Read the model definition and answer for the solid it produces. Units are mm, in the model's axes. Round coordinates to 2 decimals unless told otherwise and drop trailing zeros. Loops run counter-clockwise (first coordinate to the right, second up) from the corner with the lowest first, then second, coordinate; pieces in that order, holes last. Notation, with made-up numbers: (40.5, -31) - (77.5, -31) arc R16 cw to (77.5, 0) - close; hole circle Ø1 at (89.5, 17). An arc over 180 degrees is marked (long way). Use CSV: the item, a comma, the result in double quotes. Start each with the question number.
1. Consider line 1 along X through (y, z) = (-41, 2.55); line 2 along X through (y, z) = (-29.5, 1.7); line 3 along Y through (x, z) = (180.5, 0.3). Determine where each line is inside the solid, lowest interval first.
2. Given pin 1 Ø2.5 at (x, z) = (28, 1.5) entering from -Y; pin 2 Ø2.5 at (x, y) = (-193.01, -130.08) entering from -Z, each flat-ended and moving along its own axis, determine where each tip first touches the part or whether it passes through.
3. Find section A-A (z = 4). State how many separate pieces and enclosed holes the cut face has, and give its area (3 significant figures).
4. Find section B-B (x = -120.5). Give the vertices of the cut face in (y, z), and give its area (3 significant figures).
from build123d import *

# Parameters (mm, degrees)
SKETCH1_W           = 557
SKETCH1_H           = 150
BOSS_EXTRUDE1_DEPTH = 5
SKETCH2_W           = 30
SKETCH2_H           = 10.4
BOSS_EXTRUDE2_DEPTH = 5
SKETCH3_R           = 2.1
CUT_EXTRUDE1_DEPTH  = 10
SKETCH4_R           = 2.1
CUT_EXTRUDE2_DEPTH  = 10
SKETCH5_R           = 2.1
CUT_EXTRUDE3_DEPTH  = 10
SKETCH6_R           = 2.1
CUT_EXTRUDE4_DEPTH  = 10


with BuildPart() as part:
    # Sketch1 → Boss-Extrude1 (new body)
    with BuildSketch(Plane.XY):
        with Locations((-17.512478204, -80.075206465)):
            Rectangle(SKETCH1_W, SKETCH1_H)
    extrude(amount=BOSS_EXTRUDE1_DEPTH)

    # Sketch2 → Boss-Extrude2 (add)
    with BuildSketch(Plane.XY.offset(5)):
        with Locations((-156.762478204, -155.075206465)):
            Rectangle(SKETCH2_W, SKETCH2_H)
        with Locations((121.737521796, -155.075206465)):
            Rectangle(SKETCH2_W, SKETCH2_H)
    extrude(amount=-BOSS_EXTRUDE2_DEPTH)

    # Sketch3 → Cut-Extrude1 (cut)
    with BuildSketch(Plane.XY.offset(5)):
        with Locations((-276.012478204, -28.705206465)):
            Circle(SKETCH3_R)
        with Locations((-276.012478204, -42.775206465)):
            Circle(SKETCH3_R)
        with Locations((240.987521796, -42.775206465)):
            Circle(SKETCH3_R)
        with Locations((240.987521796, -28.705206465)):
            Circle(SKETCH3_R)
    extrude(amount=-CUT_EXTRUDE1_DEPTH, mode=Mode.SUBTRACT)

    # Sketch4 → Cut-Extrude2 (cut)
    with BuildSketch(Plane(origin=(0, 0, 0), x_dir=(-1, 0, 0), z_dir=(0, 0, -1))):
        with Locations((-240.987521796, -80.075206465)):
            Circle(SKETCH4_R)
        with Locations((276.012478204, -80.075206465)):
            Circle(SKETCH4_R)
    extrude(amount=-CUT_EXTRUDE2_DEPTH, mode=Mode.SUBTRACT)

    # Sketch5 → Cut-Extrude3 (cut)
    with BuildSketch(Plane(origin=(0, 0, 0), x_dir=(-1, 0, 0), z_dir=(0, 0, -1))):
        with Locations((-157.487521796, -130.075206465)):
            Circle(SKETCH5_R)
        with Locations((-157.487521796, -100.075206465)):
            Circle(SKETCH5_R)
    extrude(amount=-CUT_EXTRUDE3_DEPTH, mode=Mode.SUBTRACT)

    # Sketch6 → Cut-Extrude4 (cut)
    with BuildSketch(Plane(origin=(0, 0, 0), x_dir=(-1, 0, 0), z_dir=(0, 0, -1))):
        with Locations((193.012478204, -130.075206465)):
            Circle(SKETCH6_R)
        with Locations((193.012478204, -100.075206465)):
            Circle(SKETCH6_R)
    extrude(amount=-CUT_EXTRUDE4_DEPTH, mode=Mode.SUBTRACT)


solid = part.part
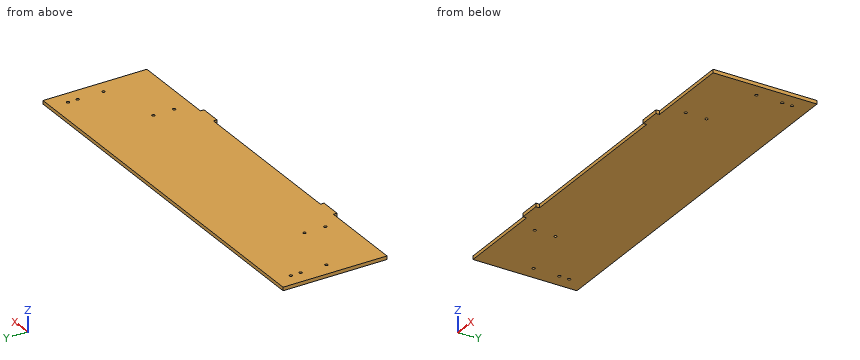
Filled sheet:
1,line 1,"x = -296.01 to -277.13, -274.89 to 239.87, 242.11 to 260.99"
1,line 2,"x = -296.01 to -277.96, -274.07 to 239.04, 242.93 to 260.99"
1,line 3,"y = -155.08 to -5.08"
2,pin 1,"stops at y = -155.08"
2,pin 2,"passes through"
3,separate pieces,"1"
3,enclosed holes,"10"
3,area,"83,700 mm²"
4,outline,"(-155.08, 0) - (-5.08, 0) - (-5.08, 5) - (-155.08, 5) - close"
4,area,"750 mm²"
